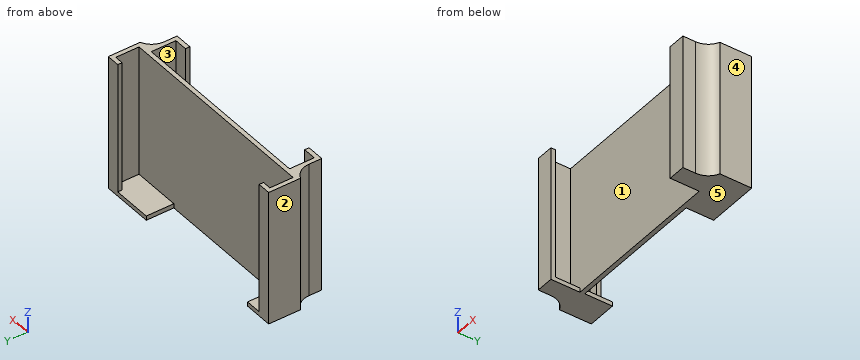
from build123d import *

# Parameters (mm, degrees)
F1_DEPTH    = 45
F2_T1_DEPTH = 45
F3_W        = 4.5
F3_H        = 8.5
F4_DEPTH    = 1.5


# Not quite as in the source:
# - a fillet or chamfer that OpenCascade refuses, or shapes differently, is made with other operations: its cross-section is extruded or revolved along the edge and cut away or added


with BuildPart() as f1:
    # F0 (on Top) → F1 (new body)
    with BuildSketch(Plane.XY):
        Polygon((36.5, 0), (0, 0), (-36.5, 0), (-36.5, 8), (-33.5, 8), (-33.5, 9.5), (-38, 9.5), (-38, -1.5), (-34.25, -1.5), (-32.75, -1.5), (0, -1.5), (32.75, -1.5), (34.25, -1.5), (38, -1.5), (38, 9.5), (33.5, 9.5), (33.5, 8), (36.5, 8), align=None)
        Polygon((-32.75, -1.5), (-34.25, -1.5), (-34.25, -11.5), (-28.25, -11.5), (-28.25, -10), (-32.75, -10), align=None)
        Polygon((34.25, -11.5), (34.25, -1.5), (32.75, -1.5), (32.75, -10), (28.25, -10), (28.25, -11.5), align=None)
    extrude(amount=F1_DEPTH)

    # F2: fillet of radius 6 on 2 edges, made by hand

    # F2_s2 → F2_t1 (join)
    with BuildSketch(Plane.XY):
        with BuildLine():
            ThreePointArc((-38, -1.5), (-35.2750628145, -3.7080468991), (-34.25, -7.0621488653))
            Line((-34.25, -7.0621488653), (-34.25, -1.5))
            Line((-34.25, -1.5), (-38, -1.5))
        make_face()
        with BuildLine():
            ThreePointArc((34.25, -7.0621488653), (35.2750628145, -3.7080468991), (38, -1.5))
            Line((38, -1.5), (34.25, -1.5))
            Line((34.25, -1.5), (34.25, -7.0621488653))
        make_face()
    extrude(amount=F2_T1_DEPTH)

    # F3 (on face) → F4 (join)
    with BuildSketch(Plane(origin=(0, 0, 0), x_dir=(1, 0, 0), z_dir=(0, 0, -1))):
        with BuildLine():
            Line((-32.75, 10), (-28.25, 10))
            Line((-28.25, 10), (-28.25, 11.5))
            Line((-28.25, 11.5), (-34.25, 11.5))
            Line((-34.25, 11.5), (-34.25, 7.0621488653))
            ThreePointArc((-34.25, 7.0621488653), (-35.2750628145, 3.7080468991), (-38, 1.5))
            Line((-38, 1.5), (-38, -9.5))
            Line((-38, -9.5), (-33.5, -9.5))
            Line((-33.5, -9.5), (-33.5, -8))
            Line((-33.5, -8), (-36.5, -8))
            Line((-36.5, -8), (-36.5, 0))
            Line((-36.5, 0), (-28, 0))
            Line((-28, 0), (20, 0))
            Line((20, 0), (36.5, 0))
            Line((36.5, 0), (36.5, -8))
            Line((36.5, -8), (33.5, -8))
            Line((33.5, -8), (33.5, -9.5))
            Line((33.5, -9.5), (38, -9.5))
            Line((38, -9.5), (38, 1.5))
            ThreePointArc((38, 1.5), (35.2750628145, 3.7080468991), (34.25, 7.0621488653))
            Line((34.25, 7.0621488653), (34.25, 11.5))
            Line((34.25, 11.5), (28.25, 11.5))
            Line((28.25, 11.5), (28.25, 10))
            Line((28.25, 10), (32.75, 10))
            Line((32.75, 10), (32.75, 1.5))
            Line((32.75, 1.5), (28.25, 1.5))
            Line((28.25, 1.5), (-28.25, 1.5))
            Line((-28.25, 1.5), (-32.75, 1.5))
            Line((-32.75, 1.5), (-32.75, 10))
        make_face()
        with Locations((-30.5, 5.75)):
            Rectangle(F3_W, F3_H)
        Polygon((-33.5, -8), (-33.5, -9.5), (-28, -9.5), (-28, 0), (-36.5, 0), (-36.5, -8), align=None)
        with Locations((30.5, 5.75)):
            Rectangle(F3_W, F3_H)
        Polygon((20, -9.5), (33.5, -9.5), (33.5, -8), (36.5, -8), (36.5, 0), (20, 0), align=None)
    extrude(amount=F4_DEPTH)


solid = f1.part
Check sheet for the modelled part. Datum: model origin and axes. Units: mm. Face numbers are marked on the shaded views. A direction names the side the tool comes from. Give positions to 0.01 mm unless a question says otherwise; leave off trailing zeros. Loops run counter-clockwise (first coordinate to the right, second up) from the corner with the lowest first, then second, coordinate; pieces in that order, holes last. Notation, with made-up numbers: M 52.25,59.5 L 79.25,59.5 A12 ccw 79.25,74.5 Z; hole C 27,64 d10. An arc over 180 degrees is marked long. Return JSON: item names as keys, results as strings. Group by question number.
1. Cross-section at B-B on z = 24. Record the boundary of the cut face in (x, y).
2. Cross-section at D-D on y = -8.5. Record the boundary of the cut face in (x, z), plus the area to 3 significant figures.
3. Go/stop test with flat-tipped pins: pin 1 (6 mm diameter, centred on x = -10, z = 11, fed in from +Y); pin 2 (3 mm diameter, centred on y = -7.5, z = 10.5, fed in from +X); pin 3 (1 mm diameter, centred on x = 9, z = 38, fed in from -Y). Record where each tip stops, or that it passes through.
4. Cross-section at A-A on y = 5. Record the boundary of the cut face in (x, z).
5. Mould release check, pull along X, two halves, no side actions. Record for the marked faces 3, 4 and 5: released by +X, released by -X, zero draft, split by the parting line, or undercut.
6. Cross-section at C-C on x = 30. Record the boundary of the cut face in (y, z), plus the area to 4 significant figures.
7. Thickness scan on L1, parallel to X at y = 1.25, z = 33.5; L2, parallel to X at y = -8.25, z = 34; L3, parallel to Z at x = -31.5, y = -6.5. Record the ranges inside material, lowest first.
8. Tool access check on the marked faces 1 and 2. Record the directions out of +Z, -Z, +X, -X, +Y, -Y that give a thin tool (end or side, any length) a straight path to the whole face; none if there is none.
Return value:
{
 "1": {"outline": "M -38,-1.5 A6 cw -34.25,-7.06 L -34.25,-11.5 L -28.25,-11.5 L -28.25,-10 L -32.75,-10 L -32.75,-1.5 L 32.75,-1.5 L 32.75,-10 L 28.25,-10 L 28.25,-11.5 L 34.25,-11.5 L 34.25,-7.06 A6 cw 38,-1.5 L 38,9.5 L 33.5,9.5 L 33.5,8 L 36.5,8 L 36.5,0 L -36.5,0 L -36.5,8 L -33.5,8 L -33.5,9.5 L -38,9.5 Z"},
 "2": {"outline": "M -34.25,-1.5 L -28.25,-1.5 L -28.25,0 L -32.75,0 L -32.75,45 L -34.25,45 Z; M 28.25,-1.5 L 34.25,-1.5 L 34.25,45 L 32.75,45 L 32.75,0 L 28.25,0 Z", "area": "153 mm^2"},
 "3": {"pin 1": "y = 0", "pin 2": "x = 34.34", "pin 3": "y = -1.5"},
 "4": {"outline": "M -38,-1.5 L -28,-1.5 L -28,0 L -36.5,0 L -36.5,45 L -38,45 Z; M 20,-1.5 L 38,-1.5 L 38,45 L 36.5,45 L 36.5,0 L 20,0 Z"},
 "5": {"face 3": "undercut", "face 4": "released by +X", "face 5": "zero draft"},
 "6": {"outline": "M -11.5,-1.5 L 9.5,-1.5 L 9.5,0 L 0,0 L 0,45 L -1.5,45 L -1.5,0 L -10,0 L -10,45 L -11.5,45 Z", "area": "166.5 mm^2"},
 "7": {"L1": "-38 to -36.5, 36.5 to 38", "L2": "-34.25 to -32.75, 32.75 to 34.25", "L3": "-1.5 to 0"},
 "8": {"face 1": "+Z", "face 2": "+Z, -Z, -X, +Y, -Y"}
}
